```python
from build123d import *

# Parameters (mm, degrees)
SKETCH1_R           = 28.5
SKETCH1_W           = 3.3
SKETCH1_H           = 8
SKETCH1_W_2         = 8
SKETCH1_H_2         = 3.3
SKETCH1_H_3         = 3.4
BOSS_EXTRUDE1_DEPTH = 5
SKETCH1_3_R         = 28.5
BOSS_EXTRUDE2_DEPTH = 40
SKETCH2_R           = 1.8
CUT_EXTRUDE1_DEPTH  = 35


with BuildPart() as part:
    # Sketch1 → Boss-Extrude1 (new body)
    with BuildSketch(Plane.XY):
        Circle(SKETCH1_R)
        with Locations((0, 16)):
            Rectangle(SKETCH1_W, SKETCH1_H, mode=Mode.SUBTRACT)
        with Locations((-16, 0)):
            Rectangle(SKETCH1_W_2, SKETCH1_H_2, mode=Mode.SUBTRACT)
        with Locations((0, -16)):
            Rectangle(SKETCH1_W, SKETCH1_H, mode=Mode.SUBTRACT)
        with Locations((16, 0)):
            Rectangle(SKETCH1_W_2, SKETCH1_H_3, mode=Mode.SUBTRACT)
    extrude(amount=BOSS_EXTRUDE1_DEPTH)


with BuildPart() as body_2:
    # Sketch1_3 → Boss-Extrude2 (new body)
    with BuildSketch(Plane.XY):
        Circle(SKETCH1_3_R)
        with BuildLine():
            Line((-5.65, 19.706026997), (-5.65, 24))
            Line((-5.65, 24), (5.65, 24))
            Line((5.65, 24), (5.65, 19.706026997))
            ThreePointArc((5.65, 19.706026997), (14.477280714, 14.514073968), (19.691622584, 5.7))
            Line((19.691622584, 5.7), (24, 5.7))
            Line((24, 5.7), (24, -5.7))
            Line((24, -5.7), (19.691622584, -5.7))
            ThreePointArc((19.691622584, -5.7), (14.477280714, -14.514073968), (5.65, -19.706026997))
            Line((5.65, -19.706026997), (5.65, -24))
            Line((5.65, -24), (-5.65, -24))
            Line((-5.65, -24), (-5.65, -19.706026997))
            ThreePointArc((-5.65, -19.706026997), (-14.495689014, -14.495689014), (-19.706026997, -5.65))
            Line((-19.706026997, -5.65), (-24, -5.65))
            Line((-24, -5.65), (-24, 5.65))
            Line((-24, 5.65), (-19.706026997, 5.65))
            ThreePointArc((-19.706026997, 5.65), (-14.495689014, 14.495689014), (-5.65, 19.706026997))
        make_face(mode=Mode.SUBTRACT)
    extrude(amount=-BOSS_EXTRUDE2_DEPTH)

    # Combine1: union part
    add(part.part)

    # Sketch2 → Cut-Extrude1 (cut, symmetric)
    with BuildSketch(Plane(origin=(0, 0, 0), x_dir=(1, 0, 0), z_dir=(0, 1, 0))):
        with Locations((0, 30)):
            Circle(SKETCH2_R)
    extrude(amount=CUT_EXTRUDE1_DEPTH, both=True, mode=Mode.SUBTRACT)


solid = body_2.part
```
Verification items for the finished model (mm, model axes). A direction names the side the tool comes from. Coordinates: 2 decimals unless noted, no trailing zeros. Loops run counter-clockwise (first coordinate to the right, second up) from the corner with the lowest first, then second, coordinate; pieces in that order, holes last. Notation, with made-up numbers: (-7.5, -19.75) -> (24.5, -19.75) arc R16 cw to (24.5, -13.75) -> close; hole circle Ø3 at (-21, 66). An arc over 180 degrees is marked (long way). Put each result on its own line as item: value.
1. Gauge pin test, flat ends, axial feed: P1, Ø10, axis at x = 17.5, z = -17, coming from the -Y side; P2, Ø3.5, axis at y = 2.5, z = -21.5, coming from the +X side; P3, Ø2.5, axis at x = 18, z = 1.5, coming from the +Y side. Record the tip position at first contact, or that the pin passes through.
Result set:
P1: stops at y = -25.61
P2: stops at x = 28.49
P3: stops at y = 23.06
2. Section check B-B, the plane y = 0. Record the boundary of the cut face in (x, z).
Result set:
outline: (-28.5, -40) -> (-24, -40) -> (-24, 0) -> (-20, 0) -> (-20, 5) -> (-28.5, 5) -> close; (-12, 0) -> (12, 0) -> (12, 5) -> (-12, 5) -> close; (20, 0) -> (24, 0) -> (24, -40) -> (28.5, -40) -> (28.5, 5) -> (20, 5) -> close
3. Section check D-D, the plane y = -14.5. Record the boundary of the cut face in (x, z).
Result set:
outline: (-24.54, -40) -> (-14.49, -40) -> (-14.49, 0) -> (-1.65, 0) -> (-1.65, 5) -> (-24.54, 5) -> close; (1.65, 0) -> (14.49, 0) -> (14.49, -40) -> (24.54, -40) -> (24.54, 5) -> (1.65, 5) -> close
4. Tool access check on faces 1 (the face through (16, 1.7, 2)), 2 (the face through (0, -24, -20)). Record the directions out of +Z, -Z, +X, -X, +Y, -Y that give a thin tool (end or side, any length) a straight path to the whole face; none if there is none.
Result set:
face 1: +Z, -Z
face 2: -Z
5. Section check A-A, the plane z = -21. Record the boundary of the cut face in (x, y), then the cut area to 3 significant figures.
Result set:
outline: circle Ø57 at (0, 0); hole (-24, -5.65) -> (-19.71, -5.65) arc R20.5 ccw to (-5.65, -19.71) -> (-5.65, -24) -> (5.65, -24) -> (5.65, -19.71) arc R20.5 ccw to (19.69, -5.7) -> (24, -5.7) -> (24, 5.7) -> (19.69, 5.7) arc R20.5 ccw to (5.65, 19.71) -> (5.65, 24) -> (-5.65, 24) -> (-5.65, 19.71) arc R20.5 ccw to (-19.71, 5.65) -> (-24, 5.65) -> close
area: 1,060 mm^2
6. Section check C-C, the plane x = 0. Record the boundary of the cut face in (y, z), then the cut area to 3 significant figures.
Result set:
outline: (-28.5, -40) -> (-24, -40) -> (-24, -31.8) -> (-28.5, -31.8) -> close; (-28.5, -28.2) -> (-24, -28.2) -> (-24, 0) -> (-20, 0) -> (-20, 5) -> (-28.5, 5) -> close; (-12, 0) -> (12, 0) -> (12, 5) -> (-12, 5) -> close; (20, 0) -> (24, 0) -> (24, -28.2) -> (28.5, -28.2) -> (28.5, 5) -> (20, 5) -> close; (24, -40) -> (28.5, -40) -> (28.5, -31.8) -> (24, -31.8) -> close
area: 533 mm^2
7. Thickness scan on line 1 (Z direction, x = 0, y = 25.65); line 2 (Z direction, x = -16.5, y = -2); line 3 (Y direction, x = -11.5, z = -4). Record the ranges inside material, lowest first.
Result set:
line 1: z = -40 to -31.8, -28.2 to 5
line 2: z = 0 to 5
line 3: y = -26.08 to -16.97, 16.97 to 26.08
